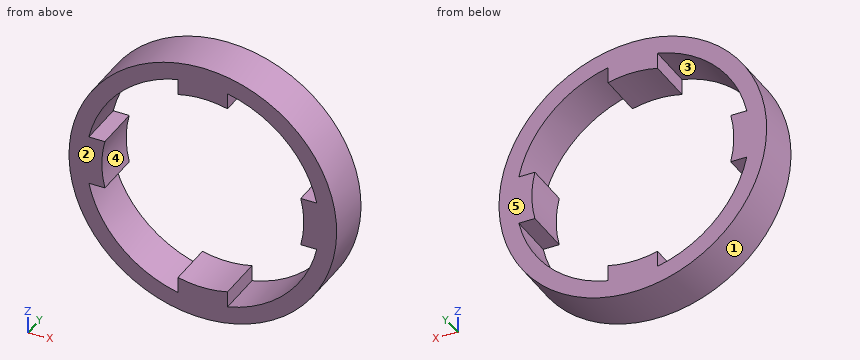
```python
from build123d import *

# Parameters (mm, degrees)
SKETCH_1_R      = 25.675
EXTRUDE_1_DEPTH = 9


with BuildPart() as part:
    # Эскиз1 → Бобышка-Вытянуть1 (new body)
    with BuildSketch(Plane(origin=(0, 0, 0), x_dir=(1, 0, 0), z_dir=(0, 1, 0))):
        with Locations(Location((0, 0, 0), (0, 0, 270))):
            Circle(SKETCH_1_R)
        with BuildLine():
            Line((-4.75, 21.864997713), (-4.75, 18.78371968))
            ThreePointArc((-4.75, 18.78371968), (0, 19.375), (4.75, 18.78371968))
            Line((4.75, 18.78371968), (4.75, 21.864997713))
            ThreePointArc((4.75, 21.864997713), (15.821514229, 15.821514229), (21.864997713, 4.75))
            Line((21.864997713, 4.75), (18.78371968, 4.75))
            ThreePointArc((18.78371968, 4.75), (19.375, 0), (18.78371968, -4.75))
            Line((18.78371968, -4.75), (21.864997713, -4.75))
            ThreePointArc((21.864997713, -4.75), (15.821514229, -15.821514229), (4.75, -21.864997713))
            Line((4.75, -21.864997713), (4.75, -18.78371968))
            ThreePointArc((4.75, -18.78371968), (0, -19.375), (-4.75, -18.78371968))
            Line((-4.75, -18.78371968), (-4.75, -21.864997713))
            ThreePointArc((-4.75, -21.864997713), (-15.821514229, -15.821514229), (-21.864997713, -4.75))
            Line((-21.864997713, -4.75), (-18.78371968, -4.75))
            ThreePointArc((-18.78371968, -4.75), (-19.375, 0), (-18.78371968, 4.75))
            Line((-18.78371968, 4.75), (-21.864997713, 4.75))
            ThreePointArc((-21.864997713, 4.75), (-15.821514229, 15.821514229), (-4.75, 21.864997713))
        make_face(mode=Mode.SUBTRACT)
    extrude(amount=EXTRUDE_1_DEPTH)


solid = part.part
```
Read the model definition and answer for the solid it produces. Units are mm, in the model's axes. Face numbers are marked on the shaded views. A direction names the side the tool comes from. Round coordinates to 2 decimals unless told otherwise and drop trailing zeros. Write each loop counter-clockwise with the first axis right and the second up, starting at its lowest first coordinate (ties: lowest second). Pieces come first, ordered by that corner, then holes. Notation, with made-up numbers: (84, -15) - (130, -15) arc R33 cw to (130, 24) - close; hole circle Ø9 at (-3.5, -15). An arc over 180 degrees is marked (long way). One line per item, written item: value.
Q1. Straight lines are drawn through the part: line 1 (X direction, y = 7, z = -20); line 2 (Z direction, x = 9.5, y = 3); line 3 (X direction, y = 7, z = 16.5). For each, find the intervals that lie inside material, in ascending order. Write a range as from..to.
The answers:
line 1: x = -16.1..-10.03, -4.75..4.75, 10.03..16.1
line 2: z = -23.85..-20.26, 20.26..23.85
line 3: x = -19.67..-15.11, 15.11..19.67
Q2. Find section C-C (z = 0). Determine the outline of the cut face in (x, y) (3 decimals), and give its area (3 significant figures).
The answers:
outline: (-25.675, 0) - (-19.375, 0) - (-19.375, 9) - (-25.675, 9) - close; (19.375, 0) - (25.675, 0) - (25.675, 9) - (19.375, 9) - close
area: 113 mm2
Q3. For a pull along X with two mould halves and no side action, classify the marked faces 1, 2 and 3 as pulls with the +X half, pulls with the -X half, needs draft (parallel to the pull), parting line crosses it, or undercut.
The answers:
face 1: parting line crosses it
face 2: needs draft
face 3: undercut
Q4. Find section B-B (y = 4.5). Determine the outline of the cut face in (x, z) (3 decimals).
The answers:
outline: circle Ø51.35 at (0, 0); hole (-21.865, -4.75) arc R22.375 ccw to (-4.75, -21.865) - (-4.75, -18.784) arc R19.375 ccw to (4.75, -18.784) - (4.75, -21.865) arc R22.375 ccw to (21.865, -4.75) - (18.784, -4.75) arc R19.375 ccw to (18.784, 4.75) - (21.865, 4.75) arc R22.375 ccw to (4.75, 21.865) - (4.75, 18.784) arc R19.375 ccw to (-4.75, 18.784) - (-4.75, 21.865) arc R22.375 ccw to (-21.865, 4.75) - (-18.784, 4.75) arc R19.375 ccw to (-18.784, -4.75) - close
Q5. Find section A-A (x = 0). Determine the outline of the cut face in (y, z) (3 decimals), and give its area (3 significant figures).
The answers:
outline: (0, -25.675) - (9, -25.675) - (9, -19.375) - (0, -19.375) - close; (0, 19.375) - (9, 19.375) - (9, 25.675) - (0, 25.675) - close
area: 113 mm2
Q6. Each of these flat-tipped pins is pushed along its axis until it touches: P1, Ø2.5, axis at x = -20, y = 5.5, coming from the -Z side; P2, Ø5, axis at y = 6, z = -8.5, coming from the +X side; P3, Ø3.5, axis at y = 3, z = 21, coming from the -X side. Where does it stop, or does it pass through?
The answers:
P1: stops at z = -17.54
P2: stops at x = 24.96
P3: stops at x = -16.99
Q7. Which of the six approach directions +Z, -Z, +X, -X, +Y, -Y give full straight-line access (tool end or side, diameter ignored) to the marked faces 4 and 5?
The answers:
face 4: +Y, -Y
face 5: +Z, -Z, +X, -X, +Y
